Verification items for the finished model (mm, model axes). Face numbers are marked on the shaded views. A direction names the side the tool comes from. Coordinates: 2 decimals unless noted, no trailing zeros. Order: outer loops, then holes, each group sorted by start corner. A loop starts at its lowest first (then second) coordinate and runs counter-clockwise, first axis right, second up. Notation, with made-up numbers: (42.25, -19) -> (55.25, -19) arc R24 cw to (55.25, 13) -> close; hole circle Ø9 at (-7.75, 65). An arc over 180 degrees is marked (long way). Write item = value, one per line. Start each with the question number.
from build123d import *

# Parameters (mm, degrees)
SKETCH1_R           = 9
BOSS_EXTRUDE2_DEPTH = 18
SKETCH2_R           = 7.5
BOSS_EXTRUDE3_DEPTH = 29
BOSS_EXTRUDE5_DEPTH = 5
SKETCH7_R           = 12.5
BOSS_EXTRUDE6_DEPTH = 18
SKETCH8_R           = 12
BOSS_EXTRUDE7_DEPTH = 29
SKETCH9_R           = 9
SKETCH9_R_2         = 7.5
CUT_EXTRUDE1_DEPTH  = 29
SKETCH10_W          = 42
SKETCH10_H          = 20
CUT_EXTRUDE2_DEPTH  = 29
CUT_EXTRUDE3_DEPTH  = 29


with BuildPart() as part:
    # Sketch1 → Boss-Extrude2 (new body, symmetric)
    with BuildSketch(Plane.XY):
        with Locations((-95, 0)):
            Circle(SKETCH1_R)
    extrude(amount=BOSS_EXTRUDE2_DEPTH, both=True)



with BuildPart() as body_2:
    # Sketch2 → Boss-Extrude3 (new body, symmetric)
    with BuildSketch(Plane.XY):
        with Locations((95, 0)):
            Circle(SKETCH2_R)
    extrude(amount=BOSS_EXTRUDE3_DEPTH, both=True)


with BuildPart() as body_3:
    # Sketch5 → Boss-Extrude5 (new body, symmetric)
    with BuildSketch(Plane(origin=(0, 0, 0), x_dir=(1, 0, 0), z_dir=(0, 1, 0))):
        Polygon((-86, -16.9), (-86, 16.897851431), (87.5, 23.242786401), (87.5, -25.734348151), align=None)
    extrude(amount=BOSS_EXTRUDE5_DEPTH, both=True)


with BuildPart() as part_1:
    add(part.part)

    add(body_3.part)  # Boss-Extrude6 merges body 3
    # Sketch7 → Boss-Extrude6 (add, symmetric)
    with BuildSketch(Plane.XY):
        with Locations((-95, 0)):
            Circle(SKETCH7_R)
    extrude(amount=BOSS_EXTRUDE6_DEPTH, both=True)


    add(body_2.part)  # Boss-Extrude7 merges body 2
    # Sketch8 → Boss-Extrude7 (add, symmetric)
    with BuildSketch(Plane.XY):
        with Locations((95, 0)):
            Circle(SKETCH8_R)
    extrude(amount=BOSS_EXTRUDE7_DEPTH, both=True)

    # Sketch9 → Cut-Extrude1 (cut, symmetric)
    with BuildSketch(Plane.XY):
        with Locations((-95, 0)):
            Circle(SKETCH9_R)
        with Locations((95, 0)):
            Circle(SKETCH9_R_2)
    extrude(amount=CUT_EXTRUDE1_DEPTH, both=True, mode=Mode.SUBTRACT)

    # Sketch10 → Cut-Extrude2 (cut, symmetric)
    with BuildSketch(Plane(origin=(0, 5, 0), x_dir=(1, 0, 0), z_dir=(0, 1, 0))):
        with Locations((86, 0)):
            Rectangle(SKETCH10_W, SKETCH10_H)
    extrude(amount=CUT_EXTRUDE2_DEPTH, both=True, mode=Mode.SUBTRACT)

    # Sketch11 → Cut-Extrude3 (cut, symmetric)
    with BuildSketch(Plane(origin=(0, 5, 0), x_dir=(1, 0, 0), z_dir=(0, 1, 0))):
        with BuildLine():
            Line((-72.828382605, 2.841663292), (-72.828382605, -3.778949024))
            ThreePointArc((-72.828382605, -3.778949024), (-71.684142411, -6.96220464), (-68.775136079, -8.688496647))
            Line((-68.775136079, -8.688496647), (-37.343188163, -14.749809861))
            ThreePointArc((-37.343188163, -14.749809861), (-30.73517362, -13.063749355), (-27.828382605, -6.894533665))
            Line((-27.828382605, -6.894533665), (-27.828382605, 5.49132779))
            ThreePointArc((-27.828382605, 5.49132779), (-30.691131262, 11.623916855), (-37.230544764, 13.367490642))
            Line((-37.230544764, 13.367490642), (-68.704733954, 7.764265074))
            ThreePointArc((-68.704733954, 7.764265074), (-71.66125077, 6.052445381), (-72.828382605, 2.841663292))
        make_face()
        with BuildLine():
            Line((-16.777023504, 0.080024287), (-16.777023504, -2.052490903))
            ThreePointArc((-16.777023504, -2.052490903), (-14.946239194, -7.145699888), (-10.291829062, -9.907767099))
            Line((-10.291829062, -9.907767099), (46.329469548, -20.826575771))
            ThreePointArc((46.329469548, -20.826575771), (54.589487728, -18.719000138), (58.222976496, -11.007480526))
            Line((58.222976496, -11.007480526), (58.222976496, 8.196063057))
            ThreePointArc((58.222976496, 8.196063057), (54.644540675, 15.861799388), (46.470273797, 18.041266623))
            Line((46.470273797, 18.041266623), (-10.179185663, 7.956187139))
            ThreePointArc((-10.179185663, 7.956187139), (-14.909612569, 5.21727563), (-16.777023504, 0.080024287))
        make_face()
    extrude(amount=CUT_EXTRUDE3_DEPTH, both=True, mode=Mode.SUBTRACT)


solid = part_1.part
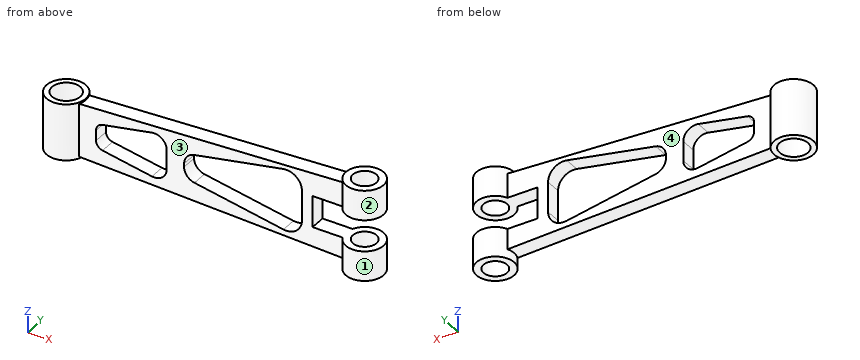
Item 1: Section check C-C (z = -21). Record the boundary of the cut face in (x, y), then the cut area to 3 significant figures.
Item 2: Section check A-A (x = -95). Record the boundary of the cut face in (y, z).
Item 3: Section check D-D (y = 0). State how many separate pieces and enclosed holes the cut face has, then the cut area to 3 significant figures.
Item 4: Gauge pin test, flat ends, axial feed: P1, Ø2.5, axis at y = 0, z = 0.5, coming from the +X side; P2, Ø4, axis at y = 9.5, z = -23, coming from the -X side; P3, Ø10, axis at x = -69, z = 5.5, coming from the -Y side. Record the tip position at first contact, or that the pin passes through.
Item 5: Section check B-B (x = 95). Record the boundary of the cut face in (y, z).
Item 6: Thickness scan on line 1 (Y direction, x = 95, z = -20); line 2 (X direction, y = 6.5, z = 17); line 3 (Y direction, x = 4, z = -19). Record the ranges inside material, lowest first.
Item 7: Mould release check, pull along X, two halves, no side actions. Record for the marked faces 1 and 2: pulls with the +X half, pulls with the -X half, needs draft (parallel to the pull), parting line crosses it, or undercut.
Item 8: Tool access check on the marked faces 3 and 4. Record the directions out of +Z, -Z, +X, -X, +Y, -Y that give a thin tool (end or side, any length) a straight path to the whole face; none if there is none.
Filled sheet:
q1.outline = (26.17, -5) -> (84.09, -5) arc R12 ccw (long way) to (84.09, 5) -> (26.17, 5) -> close; hole circle Ø15 at (95, 0)
q1.area = 848 mm^2
q2.outline = (-12.5, -18) -> (-9, -18) -> (-9, 18) -> (-12.5, 18) -> close; (9, -18) -> (12.5, -18) -> (12.5, 18) -> (9, 18) -> close
q3.separate_pieces = 4
q3.enclosed_holes = 2
q3.area = 3,960 mm^2
q4.P1 = 65
q4.P2 = 85.63
q4.P3 = -5
q5.outline = (-12, -29) -> (-7.5, -29) -> (-7.5, -10) -> (-12, -10) -> close; (-12, 10) -> (-7.5, 10) -> (-7.5, 29) -> (-12, 29) -> close; (7.5, -29) -> (12, -29) -> (12, -10) -> (7.5, -10) -> close; (7.5, 10) -> (12, 10) -> (12, 29) -> (7.5, 29) -> close
q6.line_1 = -12 to -7.5, 7.5 to 12
q6.line_2 = -105.68 to -101.22, -88.78 to -84.32, 84.91 to 91.26, 98.74 to 105.09
q6.line_3 = -5 to 5
q7.face_1 = undercut
q7.face_2 = undercut
q8.face_3 = +Z, -Z, -Y
q8.face_4 = +Z, -Z, +Y
